For this review, take the finished solid that the model builds, in its own axes (mm). A direction names the side the tool comes from. Give positions to 0.01 mm unless a question says otherwise; leave off trailing zeros. Loops run counter-clockwise (first coordinate to the right, second up) from the corner with the lowest first, then second, coordinate; pieces in that order, holes last. Notation, with made-up numbers: (64, 84.25) - (96, 84.25) arc R11 cw to (96, 89.25) - close; hole circle Ø9 at (-8.5, 40). An arc over 180 degrees is marked (long way). Answer as CSV lines item,"result".
from build123d import *

# Parameters (mm, degrees)
CYLINDER002_R     = 1
CYLINDER002_DEPTH = 1
BOX006_W          = 3
BOX006_H          = 3
BOX006_DEPTH      = 2
BOX005_W          = 3
BOX005_H          = 3
BOX005_DEPTH      = 2
BOX003_W          = 3
BOX003_H          = 3
BOX003_DEPTH      = 2
BOX004_W          = 3
BOX004_H          = 3
BOX004_DEPTH      = 2
BOX002_W          = 3
BOX002_H          = 3
BOX002_DEPTH      = 2
CYLINDER_R        = 7
CYLINDER_DEPTH    = 2
BOX_W             = 26
BOX_H             = 26
BOX_DEPTH         = 17
BOX001_W          = 30
BOX001_H          = 30
BOX001_DEPTH      = 20
CYLINDER001_R     = 3
CYLINDER001_DEPTH = 2
BOX010_W          = 6
BOX010_H          = 2
BOX010_DEPTH      = 3.4
BOX008_W          = 4
BOX008_H          = 4
BOX008_DEPTH      = 3.4
BOX007_W          = 26
BOX007_H          = 1.8
BOX007_DEPTH      = 3.4
BOX009_W          = 6
BOX009_H          = 2
BOX009_DEPTH      = 3.4
BOX011_W          = 6
BOX011_H          = 2
BOX011_DEPTH      = 3.4


with BuildPart() as obj1:
    # Cylinder002 → Cylinder002 (new body)
    with BuildSketch(Plane(origin=(0.1, 0.3, 9), x_dir=(1, 0, 0), z_dir=(0, 0, 1))):
        Circle(CYLINDER002_R)
    extrude(amount=CYLINDER002_DEPTH)


with BuildPart() as l5:
    # Box006 → Box006 (new body)
    with BuildSketch(Plane(origin=(7.67, 8.11, 7), x_dir=(1, 0, 0), z_dir=(0, 0, 1))):
        with Locations((1.5, 1.5)):
            Rectangle(BOX006_W, BOX006_H)
    extrude(amount=BOX006_DEPTH)


with BuildPart() as l4:
    # Box005 → Box005 (new body)
    with BuildSketch(Plane(origin=(3.1, 8.11, 7), x_dir=(1, 0, 0), z_dir=(0, 0, 1))):
        with Locations((1.5, 1.5)):
            Rectangle(BOX005_W, BOX005_H)
    extrude(amount=BOX005_DEPTH)


with BuildPart() as l2:
    # Box003 → Box003 (new body)
    with BuildSketch(Plane(origin=(-6.04, 8.11, 7), x_dir=(1, 0, 0), z_dir=(0, 0, 1))):
        with Locations((1.5, 1.5)):
            Rectangle(BOX003_W, BOX003_H)
    extrude(amount=BOX003_DEPTH)


with BuildPart() as l3:
    # Box004 → Box004 (new body)
    with BuildSketch(Plane(origin=(-1.47, 8.11, 7), x_dir=(1, 0, 0), z_dir=(0, 0, 1))):
        with Locations((1.5, 1.5)):
            Rectangle(BOX004_W, BOX004_H)
    extrude(amount=BOX004_DEPTH)


with BuildPart() as fusion:
    # Box002 → Box002 (new body)
    with BuildSketch(Plane(origin=(-10.61, 8.11, 7), x_dir=(1, 0, 0), z_dir=(0, 0, 1))):
        with Locations((1.5, 1.5)):
            Rectangle(BOX002_W, BOX002_H)
    extrude(amount=BOX002_DEPTH)

    # Fusion: union L5, L4, L2, L3
    add(l5.part)
    add(l4.part)
    add(l2.part)
    add(l3.part)


with BuildPart() as but:
    # Cylinder → Cylinder (new body)
    with BuildSketch(Plane(origin=(0.1, 0.3, 7), x_dir=(1, 0, 0), z_dir=(0, 0, 1))):
        Circle(CYLINDER_R)
    extrude(amount=CYLINDER_DEPTH)


with BuildPart() as maininside:
    # Box → Box (new body)
    with BuildSketch(Plane(origin=(-13, -13, -10), x_dir=(1, 0, 0), z_dir=(0, 0, 1))):
        with Locations((13, 13)):
            Rectangle(BOX_W, BOX_H)
    extrude(amount=BOX_DEPTH)


with BuildPart() as cut002:
    # Box001 → Box001 (new body)
    with BuildSketch(Plane(origin=(-15, -15, -10), x_dir=(1, 0, 0), z_dir=(0, 0, 1))):
        with Locations((15, 15)):
            Rectangle(BOX001_W, BOX001_H)
    extrude(amount=BOX001_DEPTH)

    # Cut: cut MainInside
    add(maininside.part, mode=Mode.SUBTRACT)

    # Cut001: cut But
    add(but.part, mode=Mode.SUBTRACT)

    # Cut002: cut Fusion
    add(fusion.part, mode=Mode.SUBTRACT)


with BuildPart() as cut003:
    # Cylinder001 → Cylinder001 (new body)
    with BuildSketch(Plane(origin=(0.1, 0.3, 8), x_dir=(1, 0, 0), z_dir=(0, 0, 1))):
        Circle(CYLINDER001_R)
    extrude(amount=CYLINDER001_DEPTH)

    # Fusion001: union Cut002
    add(cut002.part)

    # Cut003: cut obj1
    add(obj1.part, mode=Mode.SUBTRACT)


with BuildPart() as obj2:
    # Box010 → Box010 (new body)
    with BuildSketch(Plane(origin=(-13, 5.5, 3.6), x_dir=(1, 0, 0), z_dir=(0, 0, 1))):
        with Locations((3, 1)):
            Rectangle(BOX010_W, BOX010_H)
    extrude(amount=BOX010_DEPTH)


with BuildPart() as obj3:
    # Box008 → Box008 (new body)
    with BuildSketch(Plane(origin=(8, 0, 3.6), x_dir=(1, 0, 0), z_dir=(0, 0, 1))):
        with Locations((2, 2)):
            Rectangle(BOX008_W, BOX008_H)
    extrude(amount=BOX008_DEPTH)


with BuildPart() as obj4:
    # Box007 → Box007 (new body)
    with BuildSketch(Plane(origin=(-13, 11.2, 3.6), x_dir=(1, 0, 0), z_dir=(0, 0, 1))):
        with Locations((13, 0.9)):
            Rectangle(BOX007_W, BOX007_H)
    extrude(amount=BOX007_DEPTH)


with BuildPart() as obj5:
    # Box009 → Box009 (new body)
    with BuildSketch(Plane(origin=(-13, -4, 3.6), x_dir=(1, 0, 0), z_dir=(0, 0, 1))):
        with Locations((3, 1)):
            Rectangle(BOX009_W, BOX009_H)
    extrude(amount=BOX009_DEPTH)


with BuildPart() as fusion003:
    # Box011 → Box011 (new body)
    with BuildSketch(Plane(origin=(7, -13, 3.6), x_dir=(1, 0, 0), z_dir=(0, 0, 1))):
        with Locations((3, 1)):
            Rectangle(BOX011_W, BOX011_H)
    extrude(amount=BOX011_DEPTH)

    # Fusion002: union obj2, obj3, obj4, obj5
    add(obj2.part)
    add(obj3.part)
    add(obj4.part)
    add(obj5.part)

    # Fusion003: union Cut003
    add(cut003.part)


solid = fusion003.part
1) Insertion check: P1, Ø5, axis at x = 7, y = 4.5, coming from the -Z side; P2, Ø2.5, axis at x = -4, y = 9, coming from the -Z side; P3, Ø0.6, axis at x = 0, y = 0.5, coming from the +Z side. Each pin has a flat end and moves straight along its axis. Give the tip position at first contact, or say it passes through.
From the geometry:
P1,"stops at z = 3.6"
P2,"stops at z = 7"
P3,"stops at z = 9"
2) Consider section A-A on z = 5. Write out the cut boundary in (x, y), and give its area (3 significant figures).
From the geometry:
outline,"(-15, -15) - (15, -15) - (15, 15) - (-15, 15) - close; (8, 0) - (12, 0) - (12, 4) - (8, 4) - close; hole (-13, -13) - (7, -13) - (7, -11) - (13, -11) - (13, 11.2) - (-13, 11.2) - (-13, 7.5) - (-7, 7.5) - (-7, 5.5) - (-13, 5.5) - (-13, -2) - (-7, -2) - (-7, -4) - (-13, -4) - close"
area,"323 mm^2"
3) Consider section C-C on x = 9.75. Write out the cut boundary in (y, z), and give its area (3 significant figures).
From the geometry:
outline,"(-15, -10) - (-13, -10) - (-13, 3.6) - (-11, 3.6) - (-11, 7) - (0, 7) - (0, 3.6) - (4, 3.6) - (4, 7) - (8.11, 7) - (8.11, 9) - (11.11, 9) - (11.11, 7) - (11.2, 7) - (11.2, 3.6) - (13, 3.6) - (13, -10) - (15, -10) - (15, 10) - (-15, 10) - close"
area,"179 mm^2"
4) Consider section B-B on z = -6. Write out the cut boundary in (x, y), and give its area (3 significant figures).
From the geometry:
outline,"(-15, -15) - (15, -15) - (15, 15) - (-15, 15) - close; hole (-13, -13) - (13, -13) - (13, 13) - (-13, 13) - close"
area,"224 mm^2"
5) Consider section D-D on y = -9. Write out the cut boundary in (x, z), and give its area (3 significant figures).
From the geometry:
outline,"(-15, -10) - (-13, -10) - (-13, 7) - (13, 7) - (13, -10) - (15, -10) - (15, 10) - (-15, 10) - close"
area,"158 mm^2"
6) Draft analysis for pull direction Y (two halves, no side actions). For faces 1 (the flat face through (-4, 0, 10)), 2 (the flat face through (-10, -4, 5)), 3 (the flat face through (9, 11.11, 8)), 4 (the flat face through (0, -15, 0)), state which applies: pulls with the +Y half, pulls with the -Y half, needs draft (parallel to the pull), parting line crosses it, or undercut.
From the geometry:
face 1,"needs draft"
face 2,"undercut"
face 3,"undercut"
face 4,"pulls with the -Y half"
7) Wall thickness on line 1 (Y direction, x = 0.1, z = 9.4); line 2 (X direction, y = 8.5, z = -2.5); line 3 (Y direction, x = 0.1, z = 7.4): over which ranges is each line inside the solid? List them lowest first. Write a range as from..to.
From the geometry:
line 1,"y = -15..-0.7, 1.3..15"
line 2,"x = -15..-13, 13..15"
line 3,"y = -15..-6.7, 7.3..8.11, 11.11..15"
8) Machinability: for faces 5 (the flat face through (0, 15, 0)), 6 (the flat face through (0, 0, 9)), 7 (the flat face through (-10, -3, 3.6)), which of the approach directions +Z, -Z, +X, -X, +Y, -Y give a long, thin tool a straight path to every point of the face, cutting with its end or side? Answer none if there is none.
From the geometry:
face 5,"+Z, -Z, +X, -X, +Y"
face 6,"+Z"
face 7,"-Z"
